CAD build for the part. Positions are in the model's coordinates, mm. Round coordinates to 2 decimals unless told otherwise and drop trailing zeros. Loops run counter-clockwise (first coordinate to the right, second up) from the corner with the lowest first, then second, coordinate; pieces in that order, holes last. Notation, with made-up numbers: M 21,7.5 L 61,7.5 A5 cw 61,11.5 Z; hole C -15,-10 d1. An arc over 180 degrees is marked long. Put each result on its own line as item: value. Start each with the question number.
from build123d import *

# Parameters (mm, degrees)
SKETCH_1_R      = 250
SKETCH_1_R_2    = 115
EXTRUDE_1_DEPTH = 135
FILLET_1_R      = 67.5


with BuildPart() as part:
    # 草图1 → 凸台-拉伸1 (new body)
    with BuildSketch(Plane.XY):
        Circle(SKETCH_1_R)
        Circle(SKETCH_1_R_2, mode=Mode.SUBTRACT)
    extrude(amount=EXTRUDE_1_DEPTH)

    # 圆角1
    fillet_1_edges = [part.edges().sort_by_distance(p)[0] for p in [
        (-250, 0, 0),
        (-250, 0, 135),
        (-115, 0, 0),
        (-115, 0, 135),
    ]]
    fillet(fillet_1_edges, radius=FILLET_1_R - 0.0001)  # a hair under: the kernel refuses the full size


solid = part.part
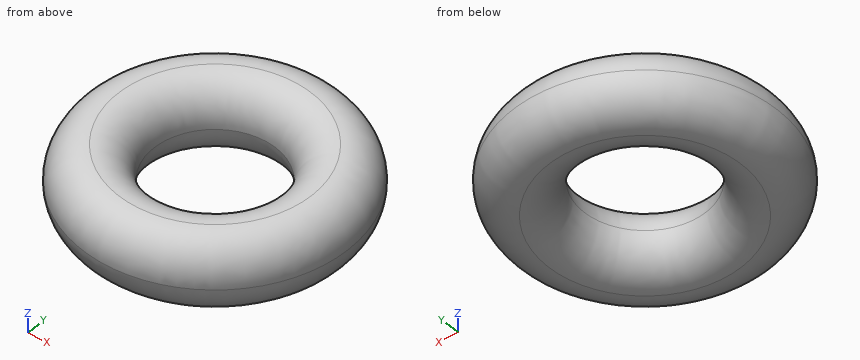
(1) Cut at D-D on z = 42.5. List the corners of the cut face in (x, y), and give its area (3 significant figures).
(2) Flat gauge pins, fed straight in: pin 1 Ø2 at (x, z) = (138, 40) entering from -Y; pin 2 Ø4 at (x, z) = (46, 91.5) entering from -Y; pin 3 Ø1.5 at (y, z) = (-176.5, 85) entering from -X; pin 4 Ø5 at (x, y) = (-50, 173) entering from +Z. Where does each tip first touch, or does it go through?
(3) Drill centre lines: line 1 along Y through (x, z) = (0, 67.55); line 2 along Y through (x, z) = (-68, 52); line 3 along X through (y, z) = (-84, 121). Where is each one in solid material? Low to high.
(4) Cut at C-C on z = 86. List the corners of the cut face in (x, y), and give its area (3 significant figures).
Taken from the geometry:
1. outline: C 0,0 d490.4; hole C 0,0 d239.6
1. area: 144,000 mm2
2. pin 1: y = -202.27
2. pin 2: y = -242.07
2. pin 3: x = -174.59
2. pin 4: z = 135
3. line 1: -250 to -115, 115 to 250
3. line 2: -238.7 to -94.97, 94.97 to 238.7
3. line 3: -207.28 to -113.67, 113.67 to 207.28
4. outline: C 0,0 d494.83; hole C 0,0 d235.17
4. area: 149,000 mm2
